Design review of the part shown in the three views and the two pictorial views. Dimensions are in mm from the part's minimum x, y and z. A direction names the side the tool comes from. Coordinates: 2 decimals unless noted, no trailing zeros. Write each loop counter-clockwise with the first axis right and the second up, starting at its lowest first coordinate (ties: lowest second). Pieces come first, ordered by that corner, then holes.
Q1. Take a section at A-A, the plane y = 4. Write out the cut boundary in (x, z).
Q2. For L1, parallel to X at y = 5, z = 27.5; L2, parallel to Y at x = 13, z = 35.2; L3, parallel to Z at x = 4.75, y = 0.75, list the stretches that pass through material, from the lowest coordinate up.
Q3. Take a section at C-C, the plane z = 32. Write out the cut boundary in (x, y).
Q4. For pin 1 Ø5 at (x, z) = (8, 15.5) entering from +Y; pin 2 Ø1.8 at (y, z) = (2.5, 27.5) entering from -X; pin 3 Ø1.5 at (x, y) = (10, 4) entering from -Z, all flat-tipped, find the tip position at first contact; note any pin that passes through.
Q5. For the marked faces 4, 5 and 6, list the 3-axis set-ups (+Z, -Z, +X, -X, +Y, -Y) from which the entire face can be reached by the end or side of a thin tool; tool diameter is ignored.
Q6. The part is to be moulded in two halves that separate along X. For the marked faces 1, 2 and 3, say which applies: released by +X, released by -X, zero draft, split by the parting line, or undercut.
Q7. Take a section at D-D, the plane x = 7. Write out the cut boundary in (y, z).
Q8. Take a section at B-B, the plane x = 13. Write out the cut boundary in (y, z), plus the area to 3 significant figures.
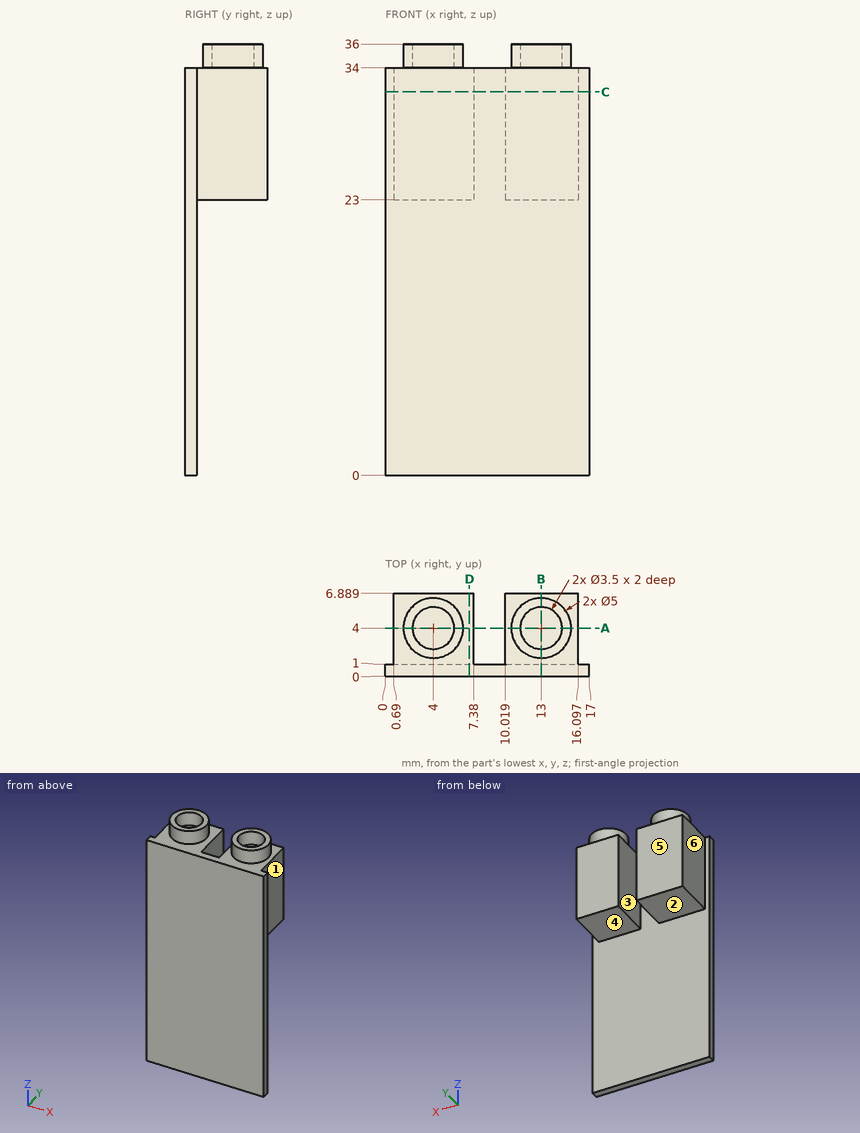
Responses:
1. outline: (0.69, 23) - (7.38, 23) - (7.38, 34) - (6.5, 34) - (6.5, 36) - (5.75, 36) - (5.75, 34) - (2.25, 34) - (2.25, 36) - (1.5, 36) - (1.5, 34) - (0.69, 34) - close; (10.02, 23) - (16.1, 23) - (16.1, 34) - (15.5, 34) - (15.5, 36) - (14.75, 36) - (14.75, 34) - (11.25, 34) - (11.25, 36) - (10.5, 36) - (10.5, 34) - (10.02, 34) - close
2. L1: x = 0.69 to 7.38, 10.02 to 16.1
2. L2: y = 1.5 to 2.25, 5.75 to 6.5
2. L3: z = 0 to 34
3. outline: (0, 0) - (17, 0) - (17, 1) - (16.1, 1) - (16.1, 6.89) - (10.02, 6.89) - (10.02, 1) - (7.38, 1) - (7.38, 6.89) - (0.69, 6.89) - (0.69, 1) - (0, 1) - close
4. pin 1: stops at y = 1
4. pin 2: stops at x = 0.69
4. pin 3: stops at z = 23
5. face 4: -Z, +X, -X, +Y
5. face 5: +Z, -Z, +X, -X, +Y
5. face 6: +Z, -Z, -X, +Y
6. face 1: released by +X
6. face 2: zero draft
6. face 3: undercut
7. outline: (0, 0) - (1, 0) - (1, 23) - (6.89, 23) - (6.89, 34) - (0, 34) - close
8. outline: (0, 0) - (1, 0) - (1, 23) - (6.89, 23) - (6.89, 34) - (6.5, 34) - (6.5, 36) - (5.75, 36) - (5.75, 34) - (2.25, 34) - (2.25, 36) - (1.5, 36) - (1.5, 34) - (0, 34) - close
8. area: 102 mm2
